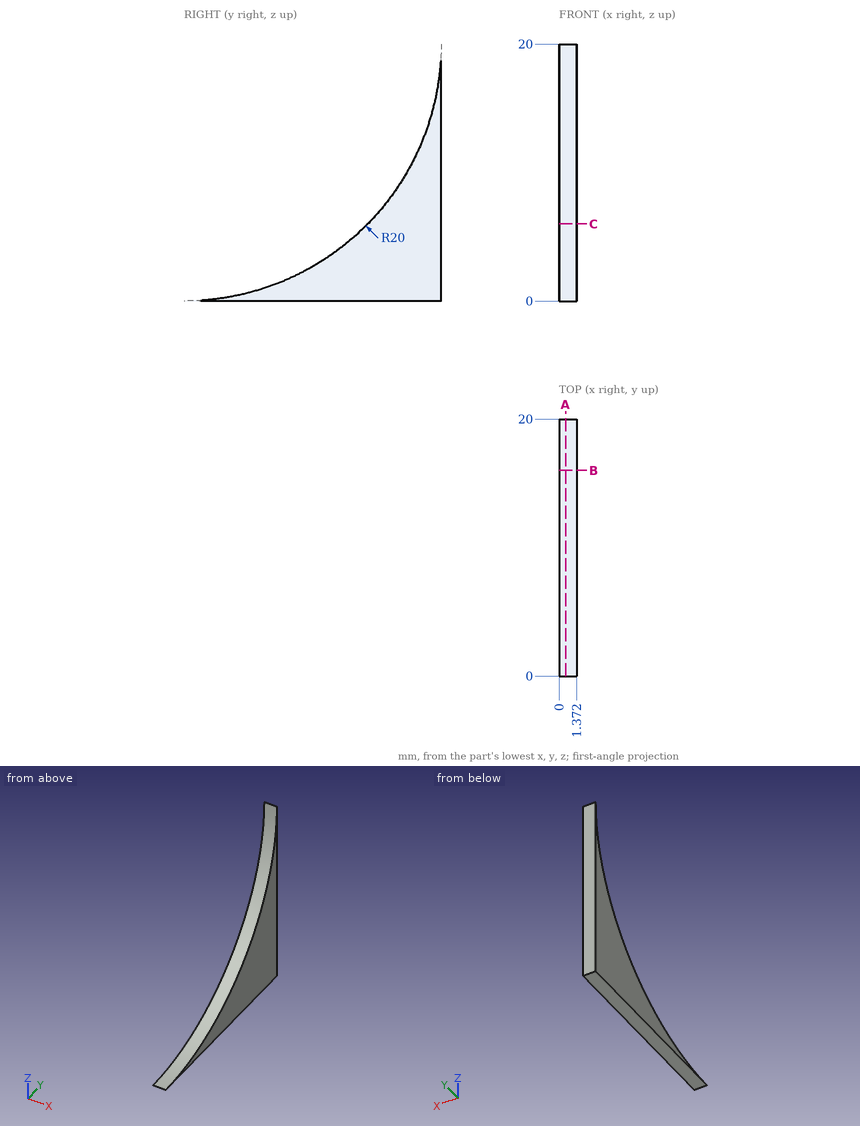
Print and shaded views of the part. All mm, measured from the part's lowest x, y and z. Coordinates: 2 decimals unless noted, no trailing zeros. Order: outer loops, then holes, each group sorted by start corner. A loop starts at its lowest first (then second) coordinate and runs counter-clockwise, first axis right, second up.
Item 1: Drill centre lines: L1, parallel to Y at x = 0.45, z = 13.75; L2, parallel to Y at x = 1.2, z = 12; L3, parallel to Z at x = 0.6, y = 6.5 (1 decimal). Where is each one in solid material? Low to high.
Filled in:
L1: y = 19 to 20
L2: y = 18.33 to 20
L3: z = 0 to 1.1
Item 2: Saw through at B-B on y = 16. List the corners of the cut face in (x, z).
Filled in:
outline: (0, 0) - (1.37, 0) - (1.37, 8) - (0, 8) - close
Item 3: Saw through at A-A on x = 0.5. List the corners of the cut face in (y, z).
Filled in:
outline: (0, 0) - (20, 0) - (20, 20) arc R20 cw to start
Item 4: Saw through at C-C on z = 6. List the corners of the cut face in (x, y).
Filled in:
outline: (0, 14.28) - (1.37, 14.28) - (1.37, 20) - (0, 20) - close
Item 5: Drop a flat-ended pin along its axis: pin 1 Ø3 at (y, z) = (10.5, 6.5) entering from -X. Give the stop position or say it passes through.
Filled in:
pin 1: passes through
